Here's how the part is built. I have some questions about the finished solid (model axes, mm). A direction names the side the tool comes from. Round coordinates to 2 decimals unless told otherwise and drop trailing zeros. Loops run counter-clockwise (first coordinate to the right, second up) from the corner with the lowest first, then second, coordinate; pieces in that order, holes last. Notation, with made-up numbers: (55.5, -5) - (66.5, -5) arc R25 ccw to (66.5, 26) - close; hole circle Ø6 at (56, 86). An arc over 180 degrees is marked (long way). Return JSON: item names as keys, results as strings. Group by question number.
```python
from build123d import *

# Parameters (mm, degrees)
SKETCH1_W           = 50.8
SKETCH1_H           = 50.8
BOSS_EXTRUDE1_DEPTH = 50.8
SKETCH2_W           = 25.4
SKETCH2_H           = 38.1
CUT_EXTRUDE1_DEPTH  = 51.8
SKETCH3_R           = 3.175
CUT_EXTRUDE2_DEPTH  = 13.7
SKETCH4_R           = 3.175
CUT_EXTRUDE3_DEPTH  = 51.8
FILLET1_R           = 12.7


with BuildPart() as part:
    # Sketch1 → Boss-Extrude1 (new body)
    with BuildSketch(Plane(origin=(0, 0, 0), x_dir=(1, 0, 0), z_dir=(0, 1, 0))):
        Rectangle(SKETCH1_W, SKETCH1_H)
    extrude(amount=BOSS_EXTRUDE1_DEPTH)

    # Sketch2 → Cut-Extrude1 (cut, through all)
    with BuildSketch(Plane(origin=(0, 50.8, 0), x_dir=(1, 0, 0), z_dir=(0, 1, 0))):
        with Locations((0, -6.35)):
            Rectangle(SKETCH2_W, SKETCH2_H)
    extrude(amount=-CUT_EXTRUDE1_DEPTH, mode=Mode.SUBTRACT)

    # Sketch3 → Cut-Extrude2 (cut, through all)
    with BuildSketch(Plane.XY.offset(-12.7)):
        with Locations((0, 25.4)):
            Circle(SKETCH3_R)
    extrude(amount=-CUT_EXTRUDE2_DEPTH, mode=Mode.SUBTRACT)

    # Sketch4 → Cut-Extrude3 (cut, through all)
    with BuildSketch(Plane(origin=(25.4, 0, 0), x_dir=(0, 0, -1), z_dir=(1, 0, 0))):
        with Locations((-12.7, 25.4)):
            Circle(SKETCH4_R)
    extrude(amount=-CUT_EXTRUDE3_DEPTH, mode=Mode.SUBTRACT)

    # Fillet1
    fillet1_edges = [part.edges().sort_by_distance(p)[0] for p in [
        (19.05, 0, 25.4),
        (19.05, 50.8, 25.4),
        (-19.05, 0, 25.4),
        (-19.05, 50.8, 25.4),
    ]]
    fillet(fillet1_edges, radius=FILLET1_R)


solid = part.part
```
Q1. Imagine slicing it at B-B, the plane y = 25.4. List the corners of the cut face in (x, z) for me (3 decimals), and give its area (3 significant figures).
Q2. For faces 1 (the flat face through (-12.7, 26, 7)), 2 (the cylindrical face through (19.14, 3.62, 21.58)), which set-ups out of +Z, -Z, +X, -X, +Y, -Y let a thin tool reach every point of the face, with its end or its side?
Q3. Imagine slicing it at A-A, the plane x = 0. List the corners of the cut face in (y, z) for me (3 decimals), and give its area (3 significant figures).
Q4. If we mould it in two halves opening along Z, with no side actions, what happens to faces 3 (the cylindrical face through (-18.96, 28.55, 13.11)), 4 (the flat face through (-19, 25, 25.4)), 5 (the flat face through (0, 31, -25.4))? For each: +Z half, -Z half, draft (parallel to the pull), parting line (faces both ways), or undercut.
Q5. Imagine slicing it at C-C, the plane z = -6. List the corners of the cut face in (x, y) for me.
Q6. Please list where these lines run through material, in increasing order: line 1 (X direction, y = 35, z = 13.5); line 2 (Y direction, x = 0, z = -18) (3 decimals); line 3 (Z direction, x = 5, y = 42.5).
Q7. Imagine slicing it at D-D, the plane x = 14.5. List the corners of the cut face in (y, z) for me (3 decimals), and give its area (3 significant figures).
Output values:
{
 "1": {"outline": "(-25.4, -25.4) - (-3.175, -25.4) - (-3.175, -12.7) - (-12.7, -12.7) - (-12.7, 9.525) - (-25.4, 9.525) - close; (-25.4, 15.875) - (-12.7, 15.875) - (-12.7, 25.4) - (-25.4, 25.4) - close; (3.175, -25.4) - (25.4, -25.4) - (25.4, 9.525) - (12.7, 9.525) - (12.7, -12.7) - (3.175, -12.7) - close; (12.7, 15.875) - (25.4, 15.875) - (25.4, 25.4) - (12.7, 25.4) - close", "area": "1,370 mm^2"},
 "2": {"face 1": "+Z, +Y, -Y", "face 2": "+Z, +X, -X, -Y"},
 "3": {"outline": "(0, -25.4) - (22.225, -25.4) - (22.225, -12.7) - (0, -12.7) - close; (28.575, -25.4) - (50.8, -25.4) - (50.8, -12.7) - (28.575, -12.7) - close", "area": "565 mm^2"},
 "4": {"face 3": "undercut", "face 4": "+Z half", "face 5": "-Z half"},
 "5": {"outline": "(-25.4, 0) - (-12.7, 0) - (-12.7, 50.8) - (-25.4, 50.8) - close; (12.7, 0) - (25.4, 0) - (25.4, 50.8) - (12.7, 50.8) - close"},
 "6": {"line 1": "x = -25.4 to -12.7, 12.7 to 25.4", "line 2": "y = 0 to 22.225, 28.575 to 50.8", "line 3": "z = -25.4 to -12.7"},
 "7": {"outline": "(0, -25.4) - (50.8, -25.4) - (50.8, 12.7) arc R12.7 ccw to (38.1, 25.4) - (12.7, 25.4) arc R12.7 ccw to (0, 12.7) - close; hole circle Ø6.35 at (25.4, 12.7)", "area": "2,480 mm^2"}
}
